For this review, take the finished solid that the model builds, in its own axes (mm). A direction names the side the tool comes from. Coordinates: 2 decimals unless noted, no trailing zeros. Write each loop counter-clockwise with the first axis right and the second up, starting at its lowest first coordinate (ties: lowest second). Pieces come first, ordered by that corner, then holes. Notation, with made-up numbers: (55, 22.25) - (68, 22.25) arc R32 cw to (68, 48.25) - close; hole circle Ø1 at (-5, -24.75). An arc over 180 degrees is marked (long way). Use one line per item in the form item = value. Start each with the question number.
1) We need section A-A (y = 38). Give the boundary of the cut face in (x, z), plus the area to 3 significant figures.
2) Mouldability with a two-part tool opening along X and no side actions: class faces 1 (the flat face through (0, 53, 32.5)), 2 (the flat face through (1, 60, 11)), 3 (the cylindrical face through (-48.794, 29.58, 25.379)) as pulls with the +X half, pulls with the -X half, needs draft (parallel to the pull), parting line crosses it, or undercut.
3) Insertion check: P1, Ø12, axis at x = 20.5, y = 43.5, coming from the +Z side; P2, Ø12, axis at x = -42, y = 29, coming from the -Z side; P3, Ø2.5, axis at x = -16.75, z = 20.5, coming from the +Y side; P4, Ø4, axis at x = -33, z = 15.5, coming from the -Y side. Each pin has a flat end and moves straight along its axis. Give the tip position at first contact, or say it passes through.
4) For L1, parallel to Z at x = -36, y = 52; L2, parallel to Z at x = -16, y = 59; L3, parallel to Y at x = 42, z = -3, list the stretches that pass through material, from the lowest coordinate up. Write a range as from..to.
5) We need section D-D (x = -24.5). Give the boundary of the cut face in (y, z), plus the area to 3 significant figures.
6) We need section C-C (x = 12). Give the boundary of the cut face in (y, z).
7) Tool access review of faces 4 (the cylindrical face through (-37.497, 43.753, -33.74)), 5 (the flat face through (-18.23, 58.48, 0.11)), 6 (the cylindrical face through (0.519, 24.65, 49.997)): name each direction out of +Z, -Z, +X, -X, +Y, -Y from which nothing blocks a thin tool from reaching the whole face with its end or side.
```python
from build123d import *

# Parameters (mm, degrees)
SKETCH_1_R          = 55
EXTRUDE_1_DEPTH     = 60
SKETCH_2_R          = 50
CUT_EXTRUDE_1_DEPTH = 50
SKETCH_3_W          = 33.5
SKETCH_3_H          = 15.4
CUT_EXTRUDE_2_DEPTH = 93.466210045
SKETCH_4_R          = 1.5
SKETCH_4_R_2        = 4
CUT_EXTRUDE_3_DEPTH = 99.234413522
CUT_EXTRUDE_4_DEPTH = 7
CHAMFER_1_SIZE      = 3


with BuildPart() as part:
    # Эскиз1 → Бобышка-Вытянуть1 (new body)
    with BuildSketch(Plane(origin=(0, 0, 0), x_dir=(1, 0, 0), z_dir=(0, 1, 0))):
        with Locations(Location((0, 0, 0), (0, 0, 270))):
            Circle(SKETCH_1_R)
    extrude(amount=EXTRUDE_1_DEPTH)

    # Эскиз2 → Вырез-Вытянуть1 (cut)
    with BuildSketch(Plane.XZ):
        with Locations(Location((0, 0, 0), (0, 0, 270))):
            Circle(SKETCH_2_R)
    extrude(amount=-CUT_EXTRUDE_1_DEPTH, mode=Mode.SUBTRACT)

    # Эскиз3 → Вырез-Вытянуть2 (cut, through all)
    with BuildSketch(Plane.XZ.offset(-50)):
        Rectangle(SKETCH_3_W, SKETCH_3_H)
    extrude(amount=-CUT_EXTRUDE_2_DEPTH, mode=Mode.SUBTRACT)

    # Эскиз4 → Вырез-Вытянуть3 (cut, through all)
    with BuildSketch(Plane(origin=(0, 60, 0), x_dir=(1, 0, 0), z_dir=(0, 1, 0))):
        with Locations(Location((-16.75, 20.5, 0), (0, 0, 270))):
            Circle(SKETCH_4_R)
        with Locations(Location((16.75, 20.5, 0), (0, 0, 270))):
            Circle(SKETCH_4_R)
        with Locations(Location((-16.75, -20.5, 0), (0, 0, 270))):
            Circle(SKETCH_4_R)
        with Locations(Location((16.75, -20.5, 0), (0, 0, 270))):
            Circle(SKETCH_4_R)
        with Locations(Location((33.591727056, -32.872418125, 0), (0, 0, 270))):
            Circle(SKETCH_4_R_2)
        with Locations(Location((-33.591727056, -32.872418125, 0), (0, 0, 270))):
            Circle(SKETCH_4_R_2)
        with Locations(Location((-33.591727056, 32.872418125, 0), (0, 0, 270))):
            Circle(SKETCH_4_R_2)
        with Locations(Location((33.591727056, 32.872418125, 0), (0, 0, 270))):
            Circle(SKETCH_4_R_2)
    extrude(amount=-CUT_EXTRUDE_3_DEPTH, mode=Mode.SUBTRACT)

    # Эскиз6 → Вырез-Вытянуть4 (cut)
    with BuildSketch(Plane.XZ.offset(-50)):
        with BuildLine():
            Line((-22.5, -32.5), (22.5, -32.5))
            ThreePointArc((22.5, -32.5), (29.571067812, -29.571067812), (32.5, -22.5))
            Line((32.5, -22.5), (32.5, 22.5))
            ThreePointArc((32.5, 22.5), (29.571067812, 29.571067812), (22.5, 32.5))
            Line((22.5, 32.5), (-22.5, 32.5))
            ThreePointArc((-22.5, 32.5), (-29.571067812, 29.571067812), (-32.5, 22.5))
            Line((-32.5, 22.5), (-32.5, -22.5))
            ThreePointArc((-32.5, -22.5), (-29.571067812, -29.571067812), (-22.5, -32.5))
        make_face()
    extrude(amount=-CUT_EXTRUDE_4_DEPTH, mode=Mode.SUBTRACT)

    # Фаска1
    chamfer_1_edges = [part.edges().sort_by_distance(p)[0] for p in [
        (-16.75, 60, 0),
    ]]
    chamfer(chamfer_1_edges, length=CHAMFER_1_SIZE - 0.0001)  # a hair under: the kernel refuses the full size


solid = part.part
```
Determined:
q1.outline = circle Ø110 at (0, 0); hole (-37.59, -32.97) arc R4 ccw to (-33.77, -36.87) arc R50 ccw to (33.77, -36.87) arc R4 ccw to (37.59, -32.97) arc R50 ccw to (37.59, 32.97) arc R4 ccw to (33.77, 36.87) arc R50 ccw to (-33.77, 36.87) arc R4 ccw to (-37.59, 32.97) arc R50 ccw to start
q1.area = 1,630 mm²
q2.face_1 = undercut
q2.face_2 = needs draft
q2.face_3 = parting line crosses it
q3.P1 = 53.05
q3.P2 = -41.58
q3.P3 = through
q3.P4 = 50
q4.L1 = -41.58..-36.07, -29.68..29.68, 36.07..41.58
q4.L2 = -52.62..-21.8, -19.2..-7.7, 7.7..19.2, 21.8..52.62
q4.L3 = 50..60
q5.outline = (0, -49.24) - (60, -49.24) - (60, 49.24) - (0, 49.24) - (0, 43.59) - (50, 43.59) - (50, 32.3) - (57, 32.3) - (57, -32.3) - (50, -32.3) - (50, -43.59) - (0, -43.59) - close
q5.area = 1,100 mm²
q6.outline = (0, -53.67) - (60, -53.67) - (60, -7.7) - (57, -7.7) - (57, -32.5) - (50, -32.5) - (50, -48.54) - (0, -48.54) - close; (0, 48.54) - (50, 48.54) - (50, 32.5) - (57, 32.5) - (57, 7.7) - (60, 7.7) - (60, 53.67) - (0, 53.67) - close
q7.face_4 = +Y, -Y
q7.face_5 = +Y
q7.face_6 = -Y
